Geometry: see drawing. Coordinates: mm, zero at the bounding-box minimum. A direction names the side the tool comes from. Coordinates: 2 decimals unless noted, no trailing zeros. Loops run counter-clockwise (first coordinate to the right, second up) from the corner with the lowest first, then second, coordinate; pieces in that order, holes last. Notation, with made-up numbers: (57.25, -37.75) - (102.25, -37.75) arc R8 ccw to (102.25, -23.75) - close; hole circle Ø6 at (78.25, 28). An arc over 180 degrees is marked (long way). Answer in a Markdown table with one row per item.
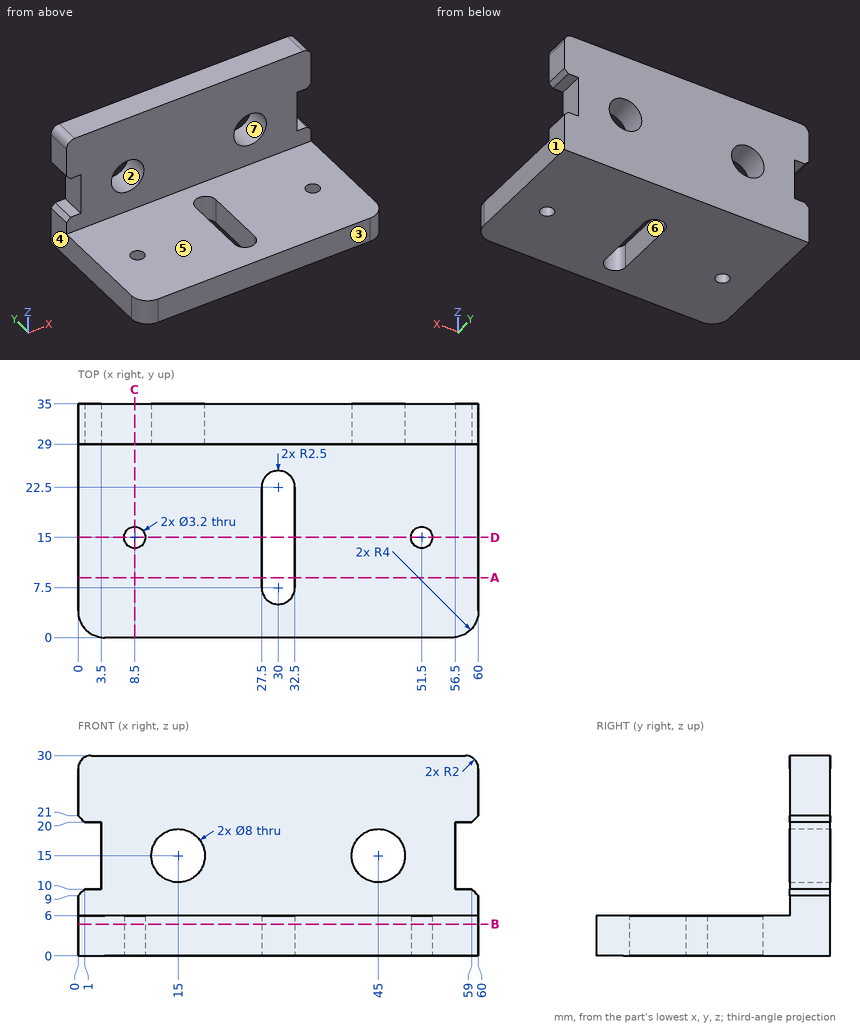
(1) First-contact query: pin 1 Ø8 at (x, y) = (21, 13.5) entering from -Z; pin 2 Ø10.5 at (x, z) = (45, 15) entering from -Y; pin 3 Ø3 at (y, z) = (31, 16) entering from +X; pin 4 Ø1.8 at (y, z) = (32.5, 13) entering from -X. Flat tips, straight axial feed; report the tip coordinate or a pass-through.
Verdict:
| item | result |
|---|---|
| pin 1 | stops at z = 0 |
| pin 2 | stops at y = 29 |
| pin 3 | stops at x = 56.5 |
| pin 4 | stops at x = 3.5 |
(2) Cut plane D-D on y = 15. Output: boundary loops of the cut face in (x, z).
Verdict:
| item | result |
|---|---|
| outline | (0, 0) - (6.9, 0) - (6.9, 6) - (0, 6) - close; (10.1, 0) - (27.5, 0) - (27.5, 6) - (10.1, 6) - close; (32.5, 0) - (49.9, 0) - (49.9, 6) - (32.5, 6) - close; (53.1, 0) - (60, 0) - (60, 6) - (53.1, 6) - close |
(3) Cut plane C-C on x = 8.5. Output: boundary loops of the cut face in (y, z), then the cut area to 3 significant figures.
Verdict:
| item | result |
|---|---|
| outline | (0, 0) - (13.4, 0) - (13.4, 6) - (0, 6) - close; (16.6, 0) - (35, 0) - (35, 30) - (29, 30) - (29, 6) - (16.6, 6) - close |
| area | 335 mm² |
(4) Pull-direction query (X, two-part tool) for the marked faces 1, 2, 3 and 4; classes: pulls with the +X half, pulls with the -X half, needs draft (parallel to the pull), parting line crosses it, or undercut.
Verdict:
| item | result |
|---|---|
| face 1 | pulls with the +X half |
| face 2 | undercut |
| face 3 | needs draft |
| face 4 | pulls with the -X half |
(5) Cut plane A-A on y = 9. Output: boundary loops of the cut face in (x, z), then the cut area to 3 significant figures.
Verdict:
| item | result |
|---|---|
| outline | (0, 0) - (27.5, 0) - (27.5, 6) - (0, 6) - close; (32.5, 0) - (60, 0) - (60, 6) - (32.5, 6) - close |
| area | 330 mm² |
(6) Ray query, probe 1 along Z at (x, y) = (15, 31.85); probe 2 along Y at (x, z) = (51.5, 4.2); probe 3 along X at (y, z) = (17.5, 1.5). Return the intervals inside material, ascending.
Verdict:
| item | result |
|---|---|
| probe 1 | z = 0 to 11, 19 to 30 |
| probe 2 | y = 0 to 13.4, 16.6 to 35 |
| probe 3 | x = 0 to 27.5, 32.5 to 60 |
(7) Access query for the marked faces 5, 6 and 7. Directions: +Z, -Z, +X, -X, +Y, -Y. A direction counts if a zero-diameter tool reaches every point of the face in a straight line with its end or side. Return the directions, or none.
Verdict:
| item | result |
|---|---|
| face 5 | +Z, +X, -X, -Y |
| face 6 | +Z, -Z |
| face 7 | +Y, -Y |
(8) Cut plane B-B on z = 4.75. Output: boundary loops of the cut face in (x, y), then the cut area to 3 significant figures.
Verdict:
| item | result |
|---|---|
| outline | (0, 4) arc R4 ccw to (4, 0) - (56, 0) arc R4 ccw to (60, 4) - (60, 35) - (0, 35) - close; hole circle Ø3.2 at (8.5, 15); hole (27.5, 7.5) arc R2.5 ccw to (32.5, 7.5) - (32.5, 22.5) arc R2.5 ccw to (27.5, 22.5) - close; hole circle Ø3.2 at (51.5, 15) |
| area | 1,980 mm² |
